```python
from build123d import *

# Parameters (mm, degrees)
SKETCH2_R                     = 15
SKETCH3_W                     = 56
SKETCH3_H                     = 56
BOSS_EXTRUDE1_DEPTH           = 6
M8_CLEARANCE_HOLE1_AT_2_COUNT = 2
M8_CLEARANCE_HOLE1_AT_2_PITCH = 56.568542495
M8_CLEARANCE_HOLE1_AT_3_COUNT = 2
M8_CLEARANCE_HOLE1_AT_3_PITCH = 40
M8_CLEARANCE_HOLE1_AT_4_COUNT = 2
M8_CLEARANCE_HOLE1_AT_4_PITCH = 40


with BuildPart() as part:
    # Sweep1: sweep along a path in Sketch1
    with BuildLine(Plane.XY) as sweep1_path:
        Line((-460, 0), (-460, 682))
        ThreePointArc((-460, 682), (-436.568542495, 738.568542495), (-380, 762))
        Line((-380, 762), (380, 762))
        ThreePointArc((380, 762), (436.568542495, 738.568542495), (460, 682))
        Line((460, 682), (460, 0))
    # Sketch2 → Sweep1 (sweep)
    with BuildSketch(Plane(origin=(0, 0, 0), x_dir=(1, 0, 0), z_dir=(0, 1, 0))):
        with Locations((-460, 0)):
            Circle(SKETCH2_R)
    sweep(path=sweep1_path.line)

    # Sketch3 → Boss-Extrude1 (add)
    with BuildSketch(Plane.XZ):
        with Locations((-460, 0)):
            Rectangle(SKETCH3_W, SKETCH3_H)
    boss_extrude1 = extrude(amount=BOSS_EXTRUDE1_DEPTH)

    # Sketch7 → M8 Clearance Hole1 (revolve, cut)
    with BuildSketch(Plane(origin=(-440, 0, 20), x_dir=(0, 0, 1), z_dir=(1, 0, 0))):
        Polygon((0, 0), (0, 25.703872786), (4.5, 23), (4.5, 0), align=None)
    m8_clearance_hole1 = revolve(axis=Axis((-440, 6.35, 20), (0, -1, 0)), mode=Mode.SUBTRACT)

    # M8 Clearance Hole1 at 2: M8 Clearance Hole1 ×2
    with Locations(*[Vector(-0.7071067811865477, 0, -0.7071067811865474) * (i * M8_CLEARANCE_HOLE1_AT_2_PITCH) for i in range(1, M8_CLEARANCE_HOLE1_AT_2_COUNT)]):
        add(m8_clearance_hole1, mode=Mode.SUBTRACT)

    # M8 Clearance Hole1 at 3: M8 Clearance Hole1 ×2
    with Locations(*[(-i * M8_CLEARANCE_HOLE1_AT_3_PITCH, 0, 0) for i in range(1, M8_CLEARANCE_HOLE1_AT_3_COUNT)]):
        add(m8_clearance_hole1, mode=Mode.SUBTRACT)

    # M8 Clearance Hole1 at 4: M8 Clearance Hole1 ×2
    with Locations(*[(0, 0, -i * M8_CLEARANCE_HOLE1_AT_4_PITCH) for i in range(1, M8_CLEARANCE_HOLE1_AT_4_COUNT)]):
        add(m8_clearance_hole1, mode=Mode.SUBTRACT)

    # Mirror1: Boss-Extrude1, M8 Clearance Hole1 across plane
    add(boss_extrude1.mirror(Plane(origin=(0, 0, 0), x_dir=(0, 0, 1), z_dir=(1, 0, 0))))
    add(m8_clearance_hole1.mirror(Plane(origin=(0, 0, 0), x_dir=(0, 0, 1), z_dir=(1, 0, 0))), mode=Mode.SUBTRACT)

    # Mirror1 copy 1 sketch → Mirror1 copy 1 (revolve, cut)
    with BuildSketch(Plane(origin=(480, 0, -20), x_dir=(0, 0, 1), z_dir=(-1, 0, 0))):
        Polygon((0, 0), (0, -25.703872786), (4.5, -23), (4.5, 0), align=None)
    revolve(axis=Axis((480, 6.35, -20), (0, 1, 0)), mode=Mode.SUBTRACT)

    # Mirror1 copy 2 sketch → Mirror1 copy 2 (revolve, cut)
    with BuildSketch(Plane(origin=(480, 0, 20), x_dir=(0, 0, 1), z_dir=(-1, 0, 0))):
        Polygon((0, 0), (0, -25.703872786), (4.5, -23), (4.5, 0), align=None)
    revolve(axis=Axis((480, 6.35, 20), (0, 1, 0)), mode=Mode.SUBTRACT)

    # Mirror1 copy 3 sketch → Mirror1 copy 3 (revolve, cut)
    with BuildSketch(Plane(origin=(440, 0, -20), x_dir=(0, 0, 1), z_dir=(-1, 0, 0))):
        Polygon((0, 0), (0, -25.703872786), (4.5, -23), (4.5, 0), align=None)
    revolve(axis=Axis((440, 6.35, -20), (0, 1, 0)), mode=Mode.SUBTRACT)


solid = part.part
```
Input: part model. Units: mm. Frame: model coordinates. A direction names the side the tool comes from. Round coordinates to 2 decimals unless told otherwise and drop trailing zeros. Order: outer loops, then holes, each group sorted by start corner. A loop starts at its lowest first (then second) coordinate and runs counter-clockwise, first axis right, second up. Notation, with made-up numbers: (-7.5, 30) - (3.5, 30) arc R17 cw to (3.5, 54) - close; hole circle Ø8 at (-2, -6). An arc over 180 degrees is marked (long way). One line per question, with ' | ' between items. Start each with the question number.
1) Cut plane C-C, the plane x = 319. Return the cut outline in (y, z).
2) Cut plane B-B, the plane y = 46. Return the cut outline in (x, z), then the cut area to 3 significant figures.
3) Cut plane A-A, the plane z = 0. Return the cut outline in (x, y).
4) Pull-direction query (X, two-part tool) for faces 3 (the flat face through (460, -6, 0)), 4 (the cylindrical face through (474.985, 336.226, -0.66)), 5 (the flat face through (448, 0, -12)); classes: +X half, -X half, draft (parallel to the pull), parting line (faces both ways), or undercut.
5) Set-up query: faces 1 (the flat face through (-448, 0, -12)), 2 (the flat face through (-460, -6, 0)). Return all of +Z, -Z, +X, -X, +Y, -Y with unobstructed straight access to the full face (end or side cutting, diameter ignored); none if empty.
6) Contact query for flat-ended pins moving along their axis: P1, Ø10.5, axis at x = 440, z = -20, coming from the -Y side; P2, Ø6, axis at y = 669, z = -1, coming from the +X side; P3, Ø12, axis at x = -317.5, z = 6.5, coming from the +Y side; P4, Ø10, axis at x = -170, z = 12, coming from the +Y side. Output: stop coordinate, or through.
7) Ray query, probe 1 along Z at (x, y) = (480, -1.2); probe 2 along X at (y, z) = (-4.3, 20); probe 3 along Y at (x, z) = (134, -0.5). Return the intervals inside material, ascending.
Worked out:
1) outline: circle Ø30 at (762, 0)
2) outline: circle Ø30 at (-460, 0); circle Ø30 at (460, 0) | area: 1,410 mm^2
3) outline: (-488, -6) - (-432, -6) - (-432, 0) - (-445, 0) - (-445, 682) arc R65 cw to (-380, 747) - (380, 747) arc R65 cw to (445, 682) - (445, 0) - (432, 0) - (432, -6) - (488, -6) - (488, 0) - (475, 0) - (475, 682) arc R95 ccw to (380, 777) - (-380, 777) arc R95 ccw to (-475, 682) - (-475, 0) - (-488, 0) - close
4) face 3: draft | face 4: undercut | face 5: undercut
5) face 1: none | face 2: +Z, -Z, +X, -X, -Y
6) P1: stops at y = -6 | P2: stops at x = 475 | P3: stops at y = 776.99 | P4: stops at y = 775.27
7) probe 1: z = -28 to -24.5, -15.5 to 15.5, 24.5 to 28 | probe 2: x = -488 to -484.5, -475.5 to -444.5, -435.5 to -432, 432 to 435.5, 444.5 to 475.5, 484.5 to 488 | probe 3: y = 747.01 to 776.99
